Input: part model. Units: mm. Frame: model coordinates. A direction names the side the tool comes from. Round coordinates to 2 decimals unless told otherwise and drop trailing zeros. Loops run counter-clockwise (first coordinate to the right, second up) from the corner with the lowest first, then second, coordinate; pieces in that order, holes last.
(1) Cut plane D-D, the plane z = 7.5. Output: boundary loops of the cut face in (x, y), and give its area (3 significant figures).
(2) Line query: line 1 (Y direction, x = 0, z = 35); line 2 (X direction, y = 8, z = 27); line 3 (Y direction, x = 0, z = 31). Output: solid intervals per line, ascending.
(3) Cut plane A-A, the plane x = 0. Output: boundary loops of the cut face in (y, z), and give its area (3 significant figures).
(4) Draft query along Y for faces 3 (the face through (0, 0, 0)), 4 (the face through (0, 0, 14)), 5 (the face through (-3.8, -17.1, 19.1)), 6 (the face through (-1.4, 10.66, 31.6)). Return one class per face: released by +Y, released by -Y, zero draft, split by the parting line, or undercut.
(5) Access query for faces 1 (the face through (-4.336, -19.524, 36.465)), 2 (the face through (4.57, 7.167, 1.972)). Directions: +Z, -Z, +X, -X, +Y, -Y. A direction counts if a zero-diameter tool reaches every point of the face in a straight line with its end or side. Return the directions, or none.
(6) First-contact query: pin 1 Ø4 at (y, z) = (1.5, 20) entering from +X; pin 2 Ø1.5 at (x, z) = (2, 13) entering from -Y; pin 3 Ø8 at (x, y) = (-7, 8.5) entering from -Z; pin 4 Ø8 at (y, z) = (-1, 21) entering from +X. Flat tips, straight axial feed; report the tip coordinate or a pass-through.
(7) Cut plane C-C, the plane z = 32.5. Output: boundary loops of the cut face in (x, y), and give its area (3 significant figures).
from build123d import *

# Parameters (mm, degrees)
F0_R     = 8.5
F1_DEPTH = 4
F2_R     = 20
F3_DEPTH = 35
F4_SIZE2 = 5
F4_SIZE  = 30
F5_R     = 7
F6_R     = 10.75
F7_DEPTH = 25
F8_SIZE  = 10


with BuildPart() as f1:
    # F0 (on Top) → F1 (new body)
    with BuildSketch(Plane.XY):
        Circle(F0_R)
    extrude(amount=F1_DEPTH)

    # F2 (on face) → F3 (join)
    with BuildSketch(Plane.XY.offset(4)):
        Circle(F2_R)
    extrude(amount=F3_DEPTH)

    # F4
    f4_edges = [f1.edges().sort_by_distance(p)[0] for p in [
        (-20, 0, 4),
    ]]
    f4_side = f1.faces().sort_by_distance((-20, 0, 21.5))[0]
    chamfer(f4_edges, length=F4_SIZE, length2=F4_SIZE2, reference=f4_side)

    # F5
    f5_edges = [f1.edges().sort_by_distance(p)[0] for p in [
        (-15, 0, 4),
    ]]
    fillet(f5_edges, radius=F5_R)

    # F6 (on face) → F7 (cut)
    with BuildSketch(Plane.XY.offset(39)):
        Circle(F6_R)
    extrude(amount=-F7_DEPTH, mode=Mode.SUBTRACT)

    # F8
    f8_edges = [f1.edges().sort_by_distance(p)[0] for p in [
        (-10.75, 0, 14),
    ]]
    chamfer(f8_edges, length=F8_SIZE)


solid = f1.part
Reported:
1. outline: circle Ø30.26 at (0, 0)
1. area: 719 mm2
2. line 1: y = -20 to -10.75, 10.75 to 20
2. line 2: x = -17.05 to -7.18, 7.18 to 17.05
2. line 3: y = -19.5 to -10.75, 10.75 to 19.5
3. outline: (-20, 34) - (-15.97, 9.85) arc R7 ccw to (-9.07, 4) - (-8.5, 4) - (-8.5, 0) - (8.5, 0) - (8.5, 4) - (9.07, 4) arc R7 ccw to (15.97, 9.85) - (20, 34) - (20, 39) - (10.75, 39) - (10.75, 24) - (0.75, 14) - (-0.75, 14) - (-10.75, 24) - (-10.75, 39) - (-20, 39) - close
3. area: 866 mm2
4. face 3: zero draft
4. face 4: undercut
4. face 5: split by the parting line
4. face 6: undercut
5. face 1: +Z, -Z
5. face 2: -Z
6. pin 1: stops at x = 17.96
6. pin 2: stops at y = -16.53
6. pin 3: stops at z = 0
6. pin 4: stops at x = 18.49
7. outline: circle Ø39.5 at (0, 0); hole circle Ø21.5 at (0, 0)
7. area: 862 mm2
